For this review, take the finished solid that the model builds, in its own axes (mm). Face numbers are marked on the shaded views. A direction names the side the tool comes from. Coordinates: 2 decimals unless noted, no trailing zeros. Order: outer loops, then holes, each group sorted by start corner. A loop starts at its lowest first (then second) coordinate and runs counter-clockwise, first axis right, second up. Notation, with made-up numbers: M -15,79 L 3,79 A11 cw 3,90 Z; hole C 30,43.25 d6. An arc over 180 degrees is marked long. Use one line per item in the form item = value. Start each with the question number.
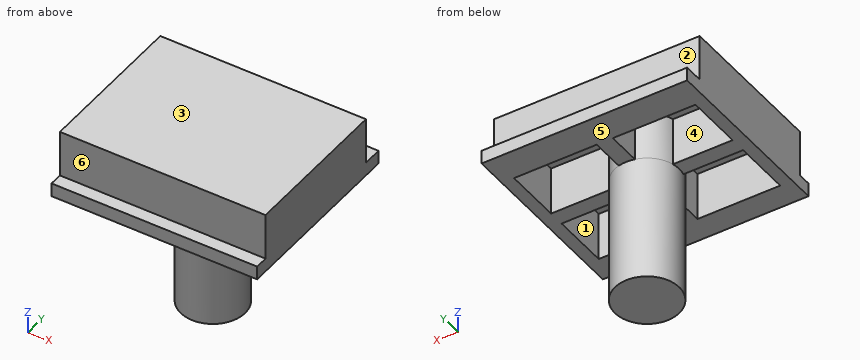
```python
from build123d import *

# Parameters (mm, degrees)
SCHIZZO1_W                   = 12.8
SCHIZZO1_H                   = 9.6
SCHIZZO1_W_2                 = 11.3
SCHIZZO1_H_2                 = 8.1
ESTRUSIONE_ESTRUSIONE1_DEPTH = 3
SCHIZZO2_W                   = 12.8
SCHIZZO2_H                   = 9.6
ESTRUSIONE_ESTRUSIONE2_DEPTH = 0.75
SCHIZZO3_W                   = 12.8
SCHIZZO3_H                   = 1.2
SCHIZZO3_H_2                 = 0.8
ESTRUSIONE_ESTRUSIONE3_DEPTH = 0.85
ESTRUSIONE_ESTRUSIONE4_DEPTH = 3
SCHIZZO5_R                   = 2
ESTRUSIONE_ESTRUSIONE5_DEPTH = 7.88


with BuildPart() as part:
    # Schizzo1 → Estrusione-Estrusione1 (new body)
    with BuildSketch(Plane.XY):
        Rectangle(SCHIZZO1_W, SCHIZZO1_H)
        Rectangle(SCHIZZO1_W_2, SCHIZZO1_H_2, mode=Mode.SUBTRACT)
    extrude(amount=ESTRUSIONE_ESTRUSIONE1_DEPTH)

    # Schizzo2 → Estrusione-Estrusione2 (add)
    with BuildSketch(Plane.XY.offset(3)):
        Rectangle(SCHIZZO2_W, SCHIZZO2_H)
    extrude(amount=ESTRUSIONE_ESTRUSIONE2_DEPTH)

    # Schizzo3 → Estrusione-Estrusione3 (add)
    with BuildSketch(Plane(origin=(0, 0, 0), x_dir=(-1, 0, 0), z_dir=(0, 0, -1))):
        with Locations((0, 5.4)):
            Rectangle(SCHIZZO3_W, SCHIZZO3_H)
        with Locations((0, -5.2)):
            Rectangle(SCHIZZO3_W, SCHIZZO3_H_2)
    extrude(amount=-ESTRUSIONE_ESTRUSIONE3_DEPTH)



with BuildPart() as body_2:
    # Schizzo4 → Estrusione-Estrusione4 (new, through all)
    with BuildSketch(Plane(origin=(0, 0, 3), x_dir=(-1, 0, 0), z_dir=(0, 0, -1))):
        with BuildLine():
            Line((5.65, -0.5), (5.65, 0.5))
            Line((5.65, 0.5), (1.936491673, 0.5))
            ThreePointArc((1.936491673, 0.5), (1.414213562, 1.414213562), (0.5, 1.936491673))
            Line((0.5, 1.936491673), (0.5, 4.05))
            Line((0.5, 4.05), (-0.5, 4.05))
            Line((-0.5, 4.05), (-0.5, 1.936491673))
            ThreePointArc((-0.5, 1.936491673), (-1.414213562, 1.414213562), (-1.936491673, 0.5))
            Line((-1.936491673, 0.5), (-5.65, 0.5))
            Line((-5.65, 0.5), (-5.65, -0.5))
            Line((-5.65, -0.5), (-1.936491673, -0.5))
            ThreePointArc((-1.936491673, -0.5), (-1.414213562, -1.414213562), (-0.5, -1.936491673))
            Line((-0.5, -1.936491673), (-0.5, -4.05))
            Line((-0.5, -4.05), (0.5, -4.05))
            Line((0.5, -4.05), (0.5, -1.936491673))
            ThreePointArc((0.5, -1.936491673), (1.414213562, -1.414213562), (1.936491673, -0.5))
            Line((1.936491673, -0.5), (5.65, -0.5))
        make_face()
    extrude(amount=ESTRUSIONE_ESTRUSIONE4_DEPTH)


with BuildPart() as part_1:
    add(part.part)

    add(body_2.part)  # Estrusione-Estrusione5 merges body 2
    # Schizzo5 → Estrusione-Estrusione5 (add)
    with BuildSketch(Plane(origin=(0, 0, 0), x_dir=(-1, 0, 0), z_dir=(0, 0, -1))):
        with Locations(Location((0, 0, 0), (0, 0, 165.522487814))):
            Circle(SCHIZZO5_R)
    extrude(amount=ESTRUSIONE_ESTRUSIONE5_DEPTH)


solid = part_1.part
```
1. Consider section C-C, the plane z = -3.5. Write out the cut boundary in (x, y).
2. To check wall thickness, follow line 1 (Y direction, x = 4.5, z = 1.5); line 2 (X direction, y = -2.25, z = 1.5); line 3 (Y direction, x = -0.5, z = -0.5). State the ranges of each line that lie inside material, in increasing order.
3. The part is to be moulded in two halves that separate along Y. For the marked faces 4, 5 and 6, say which applies: pulls with the +Y half, pulls with the -Y half, needs draft (parallel to the pull), parting line crosses it, or undercut.
4. Consider section A-A, the plane x = -2.75. Write out the cut boundary in (y, z).
5. Tool access review of the marked faces 1, 2 and 3: name each direction out of +Z, -Z, +X, -X, +Y, -Y from which nothing blocks a thin tool from reaching the whole face with its end or side.
6. For pin 1 Ø2 at (x, z) = (-2, -6.5) entering from -Y; pin 2 Ø4 at (y, z) = (-2.5, -0.5) entering from -X; pin 3 Ø3 at (x, z) = (2, -6.5) entering from -Y; pin 4 Ø1.5 at (x, z) = (-2.5, 2) entering from +Y, all flat-tipped, find the tip position at first contact; note any pin that passes through.
7. Consider section B-B, the plane y = 0. Write out the cut boundary in (x, z), plus the area to 3 significant figures.
8. Consider section D-D, the plane x = 0. Write out the cut boundary in (y, z), plus the area to 3 significant figures.
Answers follow:
q1.outline = C 0,0 d4
q2.line_1 = -4.8 to -4.05, -0.5 to 0.5, 4.05 to 4.8
q2.line_2 = -6.4 to -5.65, -0.5 to 0.5, 5.65 to 6.4
q2.line_3 = -1.94 to 1.94
q3.face_4 = undercut
q3.face_5 = needs draft
q3.face_6 = pulls with the -Y half
q4.outline = M -5.6,0 L -4.05,0 L -4.05,3 L -0.5,3 L -0.5,0 L 0.5,0 L 0.5,3 L 4.05,3 L 4.05,0 L 6,0 L 6,0.85 L 4.8,0.85 L 4.8,3.75 L -4.8,3.75 L -4.8,0.85 L -5.6,0.85 Z
q5.face_1 = -Z
q5.face_2 = +Z, +X, -X, +Y
q5.face_3 = +Z, +X, -X, +Y, -Y
q6.pin_1 = -1.73
q6.pin_2 = -6.4
q6.pin_3 = -1.94
q6.pin_4 = 4.8
q7.outline = M -6.4,0 L -2,0 L -2,-7.88 L 2,-7.88 L 2,0 L 6.4,0 L 6.4,3.75 L -6.4,3.75 Z
q7.area = 79.5 mm²
q8.outline = M -5.6,0 L -2,0 L -2,-7.88 L 2,-7.88 L 2,0 L 6,0 L 6,0.85 L 4.8,0.85 L 4.8,3.75 L -4.8,3.75 L -4.8,0.85 L -5.6,0.85 Z
q8.area = 69.2 mm²
